For this review, take the finished solid that the model builds, in its own axes (mm). Face numbers are marked on the shaded views. A direction names the side the tool comes from. Give positions to 0.01 mm unless a question says otherwise; leave off trailing zeros. Write each loop counter-clockwise with the first axis right and the second up, starting at its lowest first coordinate (ties: lowest second). Pieces come first, ordered by that corner, then holes.
1) For P1, Ø12, axis at x = -17, z = 12.5, coming from the +Y side; P2, Ø4, axis at x = -20.5, y = -2, coming from the +Z side; P3, Ø1.5, axis at x = 9, y = -3, coming from the +Z side, all flat-tipped, find the tip position at first contact; note any pin that passes through.
2) We need section C-C on z = 15. Give the boundary of the cut face in (x, y).
3) Wall thickness on line 1 along Y through (x, z) = (20.75, 1.7); line 2 along X through (y, z) = (-1.5, 2.25); line 3 along X through (y, z) = (-5, 6.75): over which ranges is each line inside the solid? List them lowest first.
4) Draft analysis for pull direction X (two halves, no side actions). For the marked faces 1, 2 and 3, state which applies: pulls with the +X half, pulls with the -X half, needs draft (parallel to the pull), parting line crosses it, or undercut.
5) We need section B-B on x = 0. Give the boundary of the cut face in (y, z).
6) We need section D-D on z = 2.5. Give the boundary of the cut face in (x, y), and give its area (3 significant figures).
7) We need section A-A on y = 0. Give the boundary of the cut face in (x, z), and give its area (3 significant figures).
8) Machinability: for the marked faces 4 and 5, which of the approach directions +Z, -Z, +X, -X, +Y, -Y give a long, thin tool a straight path to every point of the face, cutting with its end or side? Answer none if there is none.
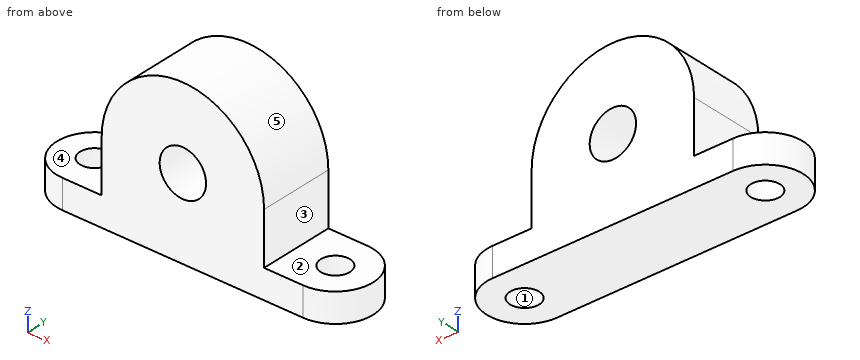
from build123d import *

# Parameters (mm, degrees)
SKETCH_1_R      = 2.5
EXTRUDE_1_DEPTH = 5
SKETCH_2_R      = 4
EXTRUDE_2_DEPTH = 13


with BuildPart() as part:
    # 草图1 → 凸台-拉伸1 (new body)
    with BuildSketch(Plane.XY):
        with BuildLine():
            Line((-20.75, -6.5), (20.75, -6.5))
            ThreePointArc((20.75, -6.5), (27.25, 0), (20.75, 6.5))
            Line((20.75, 6.5), (-20.75, 6.5))
            ThreePointArc((-20.75, 6.5), (-27.25, 0), (-20.75, -6.5))
        make_face()
        with Locations((-20.75, 0)):
            Circle(SKETCH_1_R, mode=Mode.SUBTRACT)
        with Locations((20.75, 0)):
            Circle(SKETCH_1_R, mode=Mode.SUBTRACT)
    extrude(amount=EXTRUDE_1_DEPTH)

    # 草图2 → 凸台-拉伸2 (add)
    with BuildSketch(Plane.XZ.offset(6.5)):
        with BuildLine():
            Line((-14, 14), (-14, 5))
            Line((-14, 5), (14, 5))
            Line((14, 5), (14, 14))
            ThreePointArc((14, 14), (0, 28), (-14, 14))
        make_face()
        with Locations((0, 14)):
            Circle(SKETCH_2_R, mode=Mode.SUBTRACT)
    extrude(amount=-EXTRUDE_2_DEPTH)


solid = part.part
Results list:
1. P1: stops at y = 6.5
1. P2: stops at z = 5
1. P3: stops at z = 25.31
2. outline: (-13.96, -6.5) - (-3.87, -6.5) - (-3.87, 6.5) - (-13.96, 6.5) - close; (3.87, -6.5) - (13.96, -6.5) - (13.96, 6.5) - (3.87, 6.5) - close
3. line 1: y = -6.5 to -2.5, 2.5 to 6.5
3. line 2: x = -27.07 to -22.75, -18.75 to 18.75, 22.75 to 27.07
3. line 3: x = -14 to 14
4. face 1: undercut
4. face 2: needs draft
4. face 3: pulls with the +X half
5. outline: (-6.5, 0) - (6.5, 0) - (6.5, 10) - (-6.5, 10) - close; (-6.5, 18) - (6.5, 18) - (6.5, 28) - (-6.5, 28) - close
6. outline: (-20.75, -6.5) - (20.75, -6.5) arc R6.5 ccw to (20.75, 6.5) - (-20.75, 6.5) arc R6.5 ccw to start; hole circle Ø5 at (-20.75, 0); hole circle Ø5 at (20.75, 0)
6. area: 633 mm2
7. outline: (-27.25, 0) - (-23.25, 0) - (-23.25, 5) - (-27.25, 5) - close; (-18.25, 0) - (18.25, 0) - (18.25, 5) - (14, 5) - (14, 14) arc R14 ccw to (-14, 14) - (-14, 5) - (-18.25, 5) - close; (23.25, 0) - (27.25, 0) - (27.25, 5) - (23.25, 5) - close; hole circle Ø8 at (0, 14)
7. area: 732 mm2
8. face 4: +Z, -X, +Y, -Y
8. face 5: +Z, +Y, -Y
